Source: CAD feature listing. Evaluate the final solid. Frame: model axes, mm. A direction names the side the tool comes from. Round coordinates to 2 decimals unless told otherwise and drop trailing zeros. Order: outer loops, then holes, each group sorted by start corner. A loop starts at its lowest first (then second) coordinate and runs counter-clockwise, first axis right, second up. Notation, with made-up numbers: (-8.75, 50.5) -> (10.25, 50.5) arc R21 cw to (10.25, 62.5) -> close; hole circle Ø11 at (24, 28.5). An arc over 180 degrees is marked (long way). Answer as CSV lines item,"result".
from build123d import *

# Parameters (mm, degrees)
F1_DEPTH = 609.6
F2_T     = -2.54


with BuildPart() as f1:
    # F0 (on Top) → F1 (new body)
    with BuildSketch(Plane.XY):
        Polygon((-228.6, 0), (0, 0), (0, 2133.6), (-631.449106, 1337.655261), align=None)
        Polygon((0, 2133.6), (0, 0), (228.6, 0), (631.449106, 1337.655261), align=None)
    extrude(amount=F1_DEPTH)

    # F2
    f2_openings = [f1.faces().sort_by_distance(p)[0] for p in [
        (0, 1025.524209, 609.6),
    ]]
    offset(amount=F2_T, openings=f2_openings)


solid = f1.part
1. Section query C-C on y = 1206.5. Return loops of the section in (x, z), and give its area (3 significant figures).
Results below:
outline,"(-591.95, 0) -> (591.95, 0) -> (591.95, 609.6) -> (589.3, 609.6) -> (589.3, 2.54) -> (-589.3, 2.54) -> (-589.3, 609.6) -> (-591.95, 609.6) -> close"
area,"6,230 mm2"
2. Pin query (flat end, axial travel): pin 1 (10 mm diameter, centred on x = 289.5, z = 105, fed in from +Y); pin 2 (12 mm diameter, centred on y = 378, z = 478.5, fed in from +X); pin 3 (8 mm diameter, centred on y = 1236.5, z = 365.5, fed in from -X). Return the tip coordinate at first contact, or that it passes through.
Results below:
pin 1,"y = 1774.99"
pin 2,"x = 344.25"
pin 3,"x = -602.19"
3. Section query A-A on z = 360.5. Return loops of the section in (x, y), and give its area (3 significant figures).
Results below:
outline,"(-631.45, 1337.66) -> (-228.6, 0) -> (228.6, 0) -> (631.45, 1337.66) -> (0, 2133.6) -> close; hole (-628.63, 1337.12) -> (-226.71, 2.54) -> (226.71, 2.54) -> (628.63, 1337.12) -> (0, 2129.51) -> close"
area,"13,400 mm2"
4. Line query: L1, parallel to Z at x = -288.5, y = 1738; L2, parallel to Y at x = -93, z = 474.5; L3, parallel to Y at x = -68, z = 120. Output: solid intervals per line, ascending. Write a range as [from, to].
Results below:
L1,"[0, 2.54]"
L2,"[0, 2.54], [2012.29, 2016.37]"
L3,"[0, 2.54], [2043.8, 2047.89]"
5. Reachability of faces 4 (the flat face through (-3, 0, 301)), 5 (the flat face through (-3, 2.54, 302)) from +Z, -Z, +X, -X, +Y, -Y: full face, straight path, thin tool, end or side. Return the list, or none.
Results below:
face 4,"+Z, -Z, +X, -X, -Y"
face 5,"+Z"
6. Section query B-B on x = 322.5. Return loops of the section in (y, z), and give its area (3 significant figures).
Results below:
outline,"(311.79, 0) -> (1727.09, 0) -> (1727.09, 609.6) -> (1723, 609.6) -> (1723, 2.54) -> (320.6, 2.54) -> (320.6, 609.6) -> (311.79, 609.6) -> close"
area,"11,400 mm2"
7. Mould query, pull axis Y, two halves, no side actions, for faces 1 (the flat face through (427.205, 659.464, 300.533)), 2 (the flat face through (-311.304, 1741.199, 300.533)), 3 (the flat face through (-430.487, 679.17, 301.821)). Classes: released by +Y, released by -Y, zero draft, split by the parting line, or undercut.
Results below:
face 1,"released by -Y"
face 2,"released by +Y"
face 3,"undercut"
